CAD build for the part. Positions are in the model's coordinates, mm. Face numbers are marked on the shaded views. A direction names the side the tool comes from. Round coordinates to 2 decimals unless told otherwise and drop trailing zeros. Loops run counter-clockwise (first coordinate to the right, second up) from the corner with the lowest first, then second, coordinate; pieces in that order, holes last. Notation, with made-up numbers: M 53.5,72 L 110.5,72 A29 cw 110.5,94 Z; hole C 84,25.25 d9. An arc over 180 degrees is marked long. Use a Markdown table: item, result. Add a question column.
(1) Which spindle directions (+Z, -Z, +X, -X, +Y, -Y) get a long thin tool onto all of the face, cutting with end or side? Do the marked faces 1 and 2. Say none if no direction does.
(2) Flat gauge pins, fed straight in: P1, Ø5, axis at x = 44.5, z = 35.5, coming from the +Y side; P2, Ø18, axis at x = -4.5, z = -10.5, coming from the -Y side; P3, Ø3, axis at x = -49, y = -33, coming from the +Z side. Where does each tip first touch, or does it go through?
(3) Band-saw the part on C-C, the plane z = -22.5. Write the cut outline in (x, y) (3 decimals).
(4) Wall check: L1, parallel to X at y = -36.75, z = 0 (3 decimals); L2, parallel to X at y = 2.75, z = 22.5 (3 decimals); L3, parallel to Z at x = 43, y = -32. Give the ranges that are in metal, low to high.
(5) Band-saw the part on B-B, the plane y = -9. Write the cut outline in (x, z) (3 decimals).
(6) Band-saw the part on D-D, the plane x = 43.18. Write the cut outline in (y, z) (3 decimals).
(7) Band-saw the part on A-A, the plane x = 12.57. Write the cut outline in (y, z).
from build123d import *

# Parameters (mm, degrees)
SKETCH2_W           = 95.25
SKETCH2_H           = 60
SKETCH2_R           = 2.5
BOSS_EXTRUDE1_DEPTH = 9.99998
SKETCH4_W           = 8.89
SKETCH4_H           = 60
BOSS_EXTRUDE2_DEPTH = 38.1
SKETCH6_R           = 1.5
SKETCH6_R_2         = 1.500000048
BOSS_EXTRUDE3_DEPTH = 6.35
SKETCH8_R           = 2.99974
CUT_EXTRUDE2_DEPTH  = 1.99898
CHAMFER2_SIZE       = 1.905


with BuildPart() as part:
    # Sketch2 → Boss-Extrude1 (new body)
    with BuildSketch(Plane(origin=(0, 0, 0), x_dir=(1, 0, 0), z_dir=(0, 1, 0))):
        Rectangle(SKETCH2_W, SKETCH2_H)
        with Locations(Location((12.57, 22.5, 0), (0, 0, 270))):
            Circle(SKETCH2_R, mode=Mode.SUBTRACT)
        with Locations(Location((-12.57, 22.5, 0), (0, 0, 270))):
            Circle(SKETCH2_R, mode=Mode.SUBTRACT)
        with Locations(Location((12.57, -22.5, 0), (0, 0, 270))):
            Circle(SKETCH2_R, mode=Mode.SUBTRACT)
        with Locations(Location((-12.57, -22.5, 0), (0, 0, 270))):
            Circle(SKETCH2_R, mode=Mode.SUBTRACT)
    extrude(amount=BOSS_EXTRUDE1_DEPTH)

    # Sketch4 → Boss-Extrude2 (add)
    with BuildSketch(Plane.XZ):
        with Locations((-43.18, 0)):
            Rectangle(SKETCH4_W, SKETCH4_H)
        with Locations((43.18, 0)):
            Rectangle(SKETCH4_W, SKETCH4_H)
    extrude(amount=BOSS_EXTRUDE2_DEPTH)

    # Sketch6 → Boss-Extrude3 (add)
    # profile 1 of 2: a face of its own
    with BuildSketch(Plane.XZ.offset(38.1)):
        with BuildLine():
            Line((-47.625, -4.445), (-53.34, -4.445))
            ThreePointArc((-53.34, -4.445), (-57.785, 0), (-53.34, 4.445))
            Line((-53.34, 4.445), (-47.625, 4.445))
            Line((-47.625, 4.445), (-47.625, -4.445))
        make_face()
        with Locations(Location((-53.34, 0, 0), (0, 0, 270))):
            Circle(SKETCH6_R, mode=Mode.SUBTRACT)
    # profile 2 of 2: a face of its own
    with BuildSketch(Plane.XZ.offset(38.1)):
        with BuildLine():
            Line((38.735, 30), (38.735, 35.715))
            ThreePointArc((38.735, 35.715), (43.18, 40.16), (47.625, 35.715))
            Line((47.625, 35.715), (47.625, 30))
            Line((47.625, 30), (38.735, 30))
        make_face()
        with Locations(Location((43.18, 35.715, 0), (0, 0, 270))):
            Circle(SKETCH6_R_2, mode=Mode.SUBTRACT)
    extrude(amount=-BOSS_EXTRUDE3_DEPTH)

    # Sketch8 → Cut-Extrude2 (cut)
    with BuildSketch(Plane(origin=(0, -31.75, 0), x_dir=(1, 0, 0), z_dir=(0, 1, 0))):
        with Locations(Location((43.18, -35.715, 0), (0, 0, 270))):
            Circle(SKETCH8_R)
        with Locations(Location((-53.34, 0, 0), (0, 0, 270))):
            Circle(SKETCH8_R)
    extrude(amount=-CUT_EXTRUDE2_DEPTH, mode=Mode.SUBTRACT)

    # Chamfer2
    chamfer2_edges = [part.edges().sort_by_distance(p)[0] for p in [
        (-47.625, -31.75, 0),
        (43.18, -31.75, 30),
    ]]
    chamfer(chamfer2_edges, length=CHAMFER2_SIZE)


solid = part.part
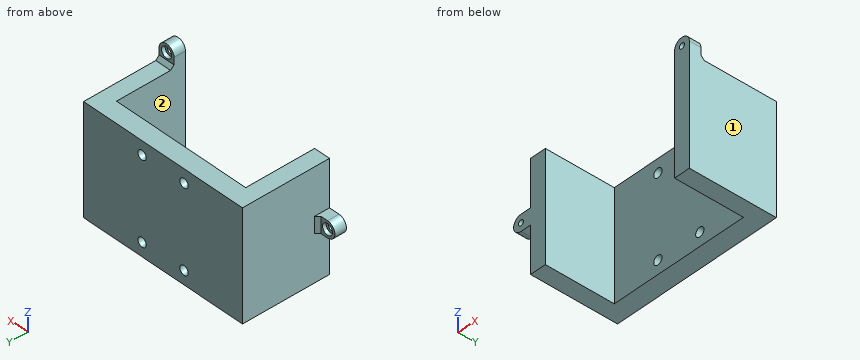
Return value:
| question | item | result |
|---|---|---|
| 1 | face 1 | +Z, -Z, +X, +Y, -Y |
| 1 | face 2 | +Z, -Z, -Y |
| 2 | P1 | y = -31.75 |
| 2 | P2 | y = 0 |
| 2 | P3 | z = 30 |
| 3 | outline | M -47.625,-38.1 L -38.735,-38.1 L -38.735,0 L -15.07,0 L -15.07,10 L -47.625,10 Z; M -10.07,0 L 10.07,0 L 10.07,10 L -10.07,10 Z; M 15.07,0 L 38.735,0 L 38.735,-38.1 L 47.625,-38.1 L 47.625,10 L 15.07,10 Z |
| 4 | L1 | -57.785 to -54.84, -51.84 to -38.735, 38.735 to 47.625 |
| 4 | L2 | -47.625 to -15.07, -10.07 to 10.07, 15.07 to 47.625 |
| 4 | L3 | -30 to 32.72, 38.71 to 40.16 |
| 5 | outline | M -47.625,-30 L -38.735,-30 L -38.735,30 L -47.625,30 Z; M 38.735,-30 L 47.625,-30 L 47.625,30 L 38.735,30 Z |
| 6 | outline | M -38.1,-30 L 10,-30 L 10,30 L -29.845,30 L -31.75,31.905 L -31.75,32.715 L -33.749,32.715 L -33.749,34.215 L -38.1,34.215 Z; M -38.1,37.215 L -33.749,37.215 L -33.749,38.715 L -31.75,38.715 L -31.75,40.16 L -38.1,40.16 Z |
| 7 | outline | M 0,-30 L 10,-30 L 10,-25 L 0,-25 Z; M 0,-20 L 10,-20 L 10,20 L 0,20 Z; M 0,25 L 10,25 L 10,30 L 0,30 Z |
